Part model, mm, in its own coordinate system. A direction names the side the tool comes from. Coordinates: 2 decimals unless noted, no trailing zeros. Write each loop counter-clockwise with the first axis right and the second up, starting at its lowest first coordinate (ties: lowest second). Pieces come first, ordered by that corner, then holes. Notation, with made-up numbers: (26, -7) - (45, -7) arc R11 cw to (45, 10) - close; hole circle Ø6 at (-32, 88.5). An arc over 180 degrees is marked (long way). Use one line per item in the form item = value. Start each with the question number.
from build123d import *

# Parameters (mm, degrees)
SKETCH_W           = 3
SKETCH_H           = 15
PAD_DEPTH          = 15
THICKNESS_T        = 1
THICKNESS_FACE2_W  = 3
THICKNESS_FACE2_H  = 15
POCKET_DEPTH       = 5
POCKET_FACE4_W     = 15
POCKET_FACE4_H     = 3
POCKET001_DEPTH    = 5
POCKET001_FACE18_W = 3
POCKET001_FACE18_H = 1
POCKET002_DEPTH    = 5


with BuildPart() as part:
    # Sketch → Pad (new body)
    with BuildSketch(Plane.XY):
        with Locations((1.5, 7.5)):
            Rectangle(SKETCH_W, SKETCH_H)
    extrude(amount=PAD_DEPTH)

    # Thickness
    thickness_openings = [part.faces().sort_by_distance(p)[0] for p in [
        (1.5, 0, 7.5),
    ]]
    offset(amount=THICKNESS_T, openings=thickness_openings)

    # Thickness Face2 → Pocket (cut)
    with BuildSketch(Plane(origin=(1.5, 15, 7.5), x_dir=(-1, 0, 0), z_dir=(0, -1, 0))):
        Rectangle(THICKNESS_FACE2_W, THICKNESS_FACE2_H)
    extrude(amount=-POCKET_DEPTH, mode=Mode.SUBTRACT)

    # Pocket Face4 → Pocket001 (cut)
    with BuildSketch(Plane(origin=(1.5, 7.5, 0), x_dir=(0, 1, 0), z_dir=(0, 0, 1))):
        Rectangle(POCKET_FACE4_W, POCKET_FACE4_H)
    extrude(amount=-POCKET001_DEPTH, mode=Mode.SUBTRACT)

    # Pocket001 Face18 → Pocket002 (cut)
    with BuildSketch(Plane(origin=(1.5, 15, -0.5), x_dir=(-1, 0, 0), z_dir=(0, -1, 0))):
        Rectangle(POCKET001_FACE18_W, POCKET001_FACE18_H)
    extrude(amount=-POCKET002_DEPTH, mode=Mode.SUBTRACT)


solid = part.part
Q1. Slice it at C-C (x = 3.6). List the corners of the cut face in (y, z), plus the area to 3 significant figures.
Q2. Which spindle directions (+Z, -Z, +X, -X, +Y, -Y) get a long thin tool onto all of the face, cutting with end or side? Do faces 5 (the cylindrical face through (1.521, 15.715, 15.699)), 6 (the flat face through (3, 8, 7)). Say none if no direction does.
Q3. Slice it at D-D (x = 1.5). List the corners of the cut face in (y, z), plus the area to 3 significant figures.
Q4. Slice it at A-A (z = 10.25). List the corners of the cut face in (x, y), plus the area to 3 significant figures.
Q5. Drill centre lines: probe 1 along X at (y, z) = (2, 6.5); probe 2 along Z at (x, y) = (0.6, 4.75); probe 3 along Z at (x, y) = (3.1, 4.25). Where is each one in solid material? Low to high.
Q6. Mould opens along X. For faces 1 (the flat face through (1, 8, 15)), 2 (the flat face through (0, 8, 7)), 3 (the flat face through (-0.2, 0, 7.4)), 4 (the cylindrical face through (3.715, 7.605, 15.699)) say: released by +X, released by -X, zero draft, split by the parting line, or undercut.
Q7. Slice it at B-B (y = 9.75). List the corners of the cut face in (x, z).
Q8. Pin check, flat tip, straight feed: P1, Ø0.9, axis at x = 1, y = 5.5, coming from the -Z side. Stop position of the tip, or through.
Solution:
q1.outline = (0, -0.8) - (15, -0.8) arc R0.8 ccw to (15.8, 0) - (15.8, 15) arc R0.8 ccw to (15, 15.8) - (0, 15.8) - close
q1.area = 262 mm2
q2.face_5 = +Z, +X, -X, +Y
q2.face_6 = -Z, +Y, -Y
q3.outline = (0, 15) - (16, 15) arc R1 ccw to (15, 16) - (0, 16) - close
q3.area = 15.8 mm2
q4.outline = (-1, 0) - (0, 0) - (0, 16) arc R1 ccw to (-1, 15) - close; (3, 0) - (4, 0) - (4, 15) arc R1 ccw to (3, 16) - close
q4.area = 31.6 mm2
q5.probe_1 = -1 to 0, 3 to 4
q5.probe_2 = 15 to 16
q5.probe_3 = -0.99 to 15.99
q6.face_1 = undercut
q6.face_2 = undercut
q6.face_3 = zero draft
q6.face_4 = released by +X
q7.outline = (-1, 0) arc R1 ccw to (0, -1) - (0, 15) - (3, 15) - (3, -1) arc R1 ccw to (4, 0) - (4, 15) arc R1 ccw to (3, 16) - (0, 16) arc R1 ccw to (-1, 15) - close
q8.P1 = 15
